The listing builds one solid part. Answer for the finished solid, in the listing's coordinates (mm). A direction names the side the tool comes from. Coordinates: 2 decimals unless noted, no trailing zeros. Loops run counter-clockwise (first coordinate to the right, second up) from the corner with the lowest first, then second, coordinate; pieces in that order, holes last. Notation, with made-up numbers: M 31.25,-19 L 35.25,-19 A23 ccw 35.25,-2 Z; hole C 1.5,82 d3. An arc over 180 degrees is marked long. Answer in a Markdown table with one row per item. Add a question column.
from build123d import *

# Parameters (mm, degrees)
BOSS_EXTRU_1_DEPTH         = 4
ESQUISSE2_W                = 2
ESQUISSE2_H                = 20
BOSS_EXTRU_2_DEPTH         = 15
ESQUISSE3_R                = 4.5
ENL_V_MAT_EXTRU_1_DEPTH    = 24
ESQUISSE4_R                = 4
ENL_V_MAT_EXTRU_2_DEPTH    = 5
R_P_TITION_LIN_AIRE1_COUNT = 2
R_P_TITION_LIN_AIRE1_PITCH = 22


with BuildPart() as part:
    # Esquisse1 → Boss.-Extru.1 (new body)
    with BuildSketch(Plane.XY):
        with BuildLine():
            Line((-2.795180723, 5.068273092), (21.204819277, 5.068273092))
            ThreePointArc((21.204819277, 5.068273092), (31.204819277, -4.931726908), (21.204819277, -14.931726908))
            Line((21.204819277, -14.931726908), (-2.795180723, -14.931726908))
            ThreePointArc((-2.795180723, -14.931726908), (-12.795180723, -4.931726908), (-2.795180723, 5.068273092))
        make_face()
    extrude(amount=BOSS_EXTRU_1_DEPTH)

    # Esquisse2 → Boss.-Extru.2 (add)
    with BuildSketch(Plane.XY):
        with Locations((9.204819277, -4.931726908)):
            Rectangle(ESQUISSE2_W, ESQUISSE2_H)
    extrude(amount=-BOSS_EXTRU_2_DEPTH)

    # Esquisse3 → Enlèv. mat.-Extru.1 (cut, through all)
    with BuildSketch(Plane(origin=(10.204819277, 0, 0), x_dir=(0, 0, -1), z_dir=(1, 0, 0))):
        with BuildLine():
            Line((15, 5.068273092), (7.792478569, 5.068273092))
            ThreePointArc((7.792478569, 5.068273092), (14.628465548, -4.931726908), (7.792478569, -14.931726908))
            Line((7.792478569, -14.931726908), (15, -14.931726908))
            Line((15, -14.931726908), (15, 5.068273092))
        make_face()
        with Locations((7.8, -4.931726908)):
            Circle(ESQUISSE3_R)
    extrude(amount=-ENL_V_MAT_EXTRU_1_DEPTH, mode=Mode.SUBTRACT)

    # Esquisse4 → Enlèv. mat.-Extru.2 (cut, through all)
    with BuildSketch(Plane(origin=(0, 0, 0), x_dir=(-1, 0, 0), z_dir=(0, 0, -1))):
        with Locations((-20.204819277, -4.931726908)):
            Circle(ESQUISSE4_R)
    enl_v_mat_extru_2 = extrude(amount=-ENL_V_MAT_EXTRU_2_DEPTH, mode=Mode.SUBTRACT)

    # Répétition linéaire1: Enlèv. mat.-Extru.2 ×2
    with Locations(*[(-i * R_P_TITION_LIN_AIRE1_PITCH, 0, 0) for i in range(1, R_P_TITION_LIN_AIRE1_COUNT)]):
        add(enl_v_mat_extru_2, mode=Mode.SUBTRACT)


solid = part.part
(1) A cutting plane is placed at A-A (x = 19.5). Give the vertices of the cut face in (y, z).
(2) Each of these flat-tipped pins is pushed along its axis until it touches: pin 1 (6 mm diameter, centred on x = 0.5, z = -2.5, fed in from -Y); pin 2 (7 mm diameter, centred on x = -1.8, y = -4.93, fed in from -Z); pin 3 (6 mm diameter, centred on x = 16, y = -5.5, fed in from -Z). Where does it stop, or does it pass through?
(3) For faces 1 (the face through (10.205, -5, -2)), 2 (the face through (8.205, -5, -2)), 3 (the face through (9, -14.932, 1)), determine the directions among +Z, -Z, +X, -X, +Y, -Y from which every point of the face is accessible in a straight line to the end or side of a thin tool.
(4) Straight lines are drawn through the part: line 1 (Y direction, x = 9.7, z = -7.8); line 2 (X direction, y = -6.25, z = -3); line 3 (Z direction, x = 5, y = -5.25). For each, find the intervals that lie inside material, in ascending order.
(5) A cutting plane is placed at B-B (y = -8). Give the vertices of the cut face in (x, z), plus the area to 3 significant figures.
(6) The mould has two halves that part along X. Classify faces 4 (the face through (9.219, -4.752, -14.627)), 5 (the face through (16.4, -3.7, 2)), 6 (the face through (1.379, -7.366, 1.972)), 7 (the face through (-12.793, -5.152, 1.972)): released by +X, released by -X, zero draft, split by the parting line, or undercut.
(7) A cutting plane is placed at D-D (y = 3.75). Give the vertices of the cut face in (x, z), plus the area to 3 significant figures.
(8) A cutting plane is placed at C-C (z = -2). Give the vertices of the cut face in (x, y), plus the area to 3 significant figures.
Solved:
| question | item | result |
|---|---|---|
| 1 | outline | M -14.93,0 L -8.87,0 L -8.87,4 L -14.93,4 Z; M -0.99,0 L 5.07,0 L 5.07,4 L -0.99,4 Z |
| 2 | pin 1 | stops at y = -14.93 |
| 2 | pin 2 | passes through |
| 2 | pin 3 | stops at z = 0 |
| 3 | face 1 | -Z, +X, +Y, -Y |
| 3 | face 2 | -Z, -X, +Y, -Y |
| 3 | face 3 | +Z, -Z, +X, -X, -Y |
| 4 | line 1 | y = -14.93 to -9.43, -0.43 to 5.07 |
| 4 | line 2 | x = 8.2 to 10.2 |
| 4 | line 3 | z = 0 to 4 |
| 5 | outline | M -12.31,0 L -4.36,0 L -4.36,4 L -12.31,4 Z; M 0.77,0 L 8.2,0 L 8.2,-4.51 L 10.2,-4.51 L 10.2,0 L 17.64,0 L 17.64,4 L 0.77,4 Z; M 8.2,-14.18 L 10.2,-14.18 L 10.2,-11.09 L 8.2,-11.09 Z; M 22.77,0 L 30.72,0 L 30.72,4 L 22.77,4 Z |
| 5 | area | 146 mm² |
| 6 | face 4 | zero draft |
| 6 | face 5 | undercut |
| 6 | face 6 | undercut |
| 6 | face 7 | released by -X |
| 7 | outline | M -7.76,0 L 8.2,0 L 8.2,-10.21 L 10.2,-10.21 L 10.2,0 L 26.17,0 L 26.17,4 L -7.76,4 Z |
| 7 | area | 156 mm² |
| 8 | outline | M 8.2,-14.93 L 10.2,-14.93 L 10.2,5.07 L 8.2,5.07 Z |
| 8 | area | 40.0 mm² |
